Verification items for the finished model (mm, model axes). A direction names the side the tool comes from. Give positions to 0.01 mm unless a question says otherwise; leave off trailing zeros. Order: outer loops, then holes, each group sorted by start corner. A loop starts at its lowest first (then second) coordinate and runs counter-clockwise, first axis right, second up. Notation, with made-up numbers: M 59.25,-3 L 109.25,-3 A35 ccw 109.25,34 Z; hole C 38.25,31.5 d1. An arc over 180 degrees is marked long. Answer as a JSON object with one key per item and string values.
Autodesk Inventor part; units mm, degrees
ref_plane "YZ Plane" through (0, 0, 0) normal (1, 0, 0) x (0, 1, 0)
ref_plane "XZ Plane" through (0, 0, 0) normal (0, 1, 0) x (-1, 0, 0)
ref_plane "XY Plane" through (0, 0, 0) normal (0, 0, 1) x (1, 0, 0)
sketch "Sketch1" plane through (0, 0, 0) normal (0, 1, 0) x (-1, 0, 0)
  line L0 (0, 0) -> (-94, 0)
  line L1 (-94, 0) -> (-94, -34)
  line L2 (-94, -34) -> (0, -34)
  line L3 (0, -34) -> (0, 0)
  dimension "d0" = 34
  dimension "d1" = 94
extrude "Extrusion1" add sketch "Sketch1" along normal blind 35
sketch "Sketch2" plane through (0, 35, 0) normal (0, 1, 0) x (1, 0, 0)
  line L0 (35.0106, 7.0576) -> (60.2075, 7.0576)
  line L1 (60.2075, 7.0576) -> (60.2075, 10.8183)
  line L2 (60.2075, 10.8183) -> (35.0106, 10.8183)
  line L3 (35.0106, 10.8183) -> (35.0106, 7.0576)
  line L4 (35.0106, 7.0576) -> (39.3355, 7.0576)
  line L5 (39.3355, 7.0576) -> (39.3355, 22.8526)
  line L6 (39.3355, 22.8526) -> (35.0106, 22.8526)
  line L7 (35.0106, 22.8526) -> (35.0106, 7.0576)
  line L8 (35.0106, 22.8526) -> (60.2075, 22.8526)
  line L9 (60.2075, 22.8526) -> (60.2075, 19.0919)
  line L10 (60.2075, 19.0919) -> (35.0106, 19.0919)
  line L11 (35.0106, 19.0919) -> (35.0106, 22.8526)
  line L12 (60.2075, 22.8526) -> (56.0707, 22.8526)
  line L13 (56.0707, 22.8526) -> (56.0707, 7.0576)
  line L14 (56.0707, 7.0576) -> (60.2075, 7.0576)
  line L15 (60.2075, 7.0576) -> (60.2075, 22.8526)
  line L16 (46.1048, 7.0576) -> (50.2416, 7.0576)
  line L17 (50.2416, 7.0576) -> (50.2416, 22.8526)
  line L18 (50.2416, 22.8526) -> (46.1048, 22.8526)
  line L19 (46.1048, 22.8526) -> (46.1048, 7.0576)
  point P0 (0, 0)
  point P1 (39.3355, 10.8183)
  point P2 (39.3355, 19.0919)
  point P3 (46.1048, 19.0919)
  point P4 (46.1048, 10.8183)
  point P5 (50.2416, 19.0919)
  point P6 (56.0707, 19.0919)
  point P7 (56.0707, 10.8183)
  point P8 (50.2416, 10.8183)
extrude "Extrusion2" add sketch "Sketch2" along normal blind 2 contours L3 L2 L5 L0 | L5 L2 L19 L0 | L7 L10 L5 L2 | L19 L2 L17 L0 | L7 L6 L5 L10 | L17 L2 L13 L0 | L19 L10 L17 L2 | L5 L8 L19 L10 | L13 L2 L1 L0 | L19 L8 L17 L10 | L13 L10 L15 L2 | L17 L8 L13 L10 | L13 L8 L9 L10
properties part number "Battery Lipo"
Q1. Gauge pin test, flat ends, axial feed: pin 1 Ø1.6 at (y, z) = (36.5, -18.5) entering from -X; pin 2 Ø8 at (x, y) = (53.5, 7.5) entering from +Z; pin 3 Ø0.6 at (y, z) = (36, -14) entering from +X; pin 4 Ø1.5 at (x, z) = (15, -26) entering from +Y. Record the tip position at first contact, or that the pin passes through.
Resolved:
{"pin 1": "stops at x = 35.01", "pin 2": "stops at z = 0", "pin 3": "stops at x = 60.21", "pin 4": "stops at y = 35"}
Q2. Tool access check on faces 1 (the face through (39.336, 36, -15)), 2 (the face through (47, 36, -7.058)), 3 (the face through (60.208, 36, -15)), 4 (the face through (35.011, 36, -15)). Record the directions out of +Z, -Z, +X, -X, +Y, -Y that give a thin tool (end or side, any length) a straight path to the whole face; none if there is none.
Resolved:
{"face 1": "+Y", "face 2": "+Z, +X, -X, +Y", "face 3": "+Z, -Z, +X, +Y", "face 4": "+Z, -Z, -X, +Y"}
Q3. Section check D-D on x = 28.5. Record the cut outline in (y, z).
Resolved:
{"outline": "M 0,-34 L 35,-34 L 35,0 L 0,0 Z"}
Q4. Section check A-A on z = -9. Record the cut outline in (x, y), then the cut area to 3 significant figures.
Resolved:
{"outline": "M 0,0 L 94,0 L 94,35 L 60.21,35 L 60.21,37 L 35.01,37 L 35.01,35 L 0,35 Z", "area": "3,340 mm²"}
Q5. Section check C-C on z = -24. Record the cut outline in (x, y), then the cut area to 3 significant figures.
Resolved:
{"outline": "M 0,0 L 94,0 L 94,35 L 0,35 Z", "area": "3,290 mm²"}
Q6. Section check B-B on x = 43.5. Record the cut outline in (y, z).
Resolved:
{"outline": "M 0,-34 L 35,-34 L 35,-22.85 L 37,-22.85 L 37,-19.09 L 35,-19.09 L 35,-10.82 L 37,-10.82 L 37,-7.06 L 35,-7.06 L 35,0 L 0,0 Z"}
Q7. Release check for a two-part mould opening along Z. For faces 5 (the face through (43, 36, -10.818)), 6 (the face through (47, 37, -15)), 7 (the face through (48, 36, -22.853)) record: +Z half, -Z half, draft (parallel to the pull), parting line (faces both ways), or undercut.
Resolved:
{"face 5": "undercut", "face 6": "draft", "face 7": "-Z half"}
Q8. Material ranges on L1, parallel to Y at x = 13, z = -5, recorded low to high.
Resolved:
{"L1": "y = 0 to 35"}
